The model under review builds one solid part; all positions refer to its coordinate system, in mm. A direction names the side the tool comes from. Round coordinates to 2 decimals unless told otherwise and drop trailing zeros. Order: outer loops, then holes, each group sorted by start corner. A loop starts at its lowest first (then second) coordinate and runs counter-clockwise, first axis right, second up. Notation, with made-up numbers: (26.5, 48) -> (42.5, 48) arc R22 cw to (42.5, 60) -> close; hole circle Ø11 at (32, -31). An arc over 180 degrees is marked (long way). Use a Markdown table: item, result. Add a question column.
```python
from build123d import *

# Parameters (mm, degrees)
CUT_EXTRUDE_1_DEPTH = 1.5
CHAMFER_1_SIZE      = 0.2


with BuildPart() as part:
    # 草图1 → 旋转1 (revolve)
    with BuildSketch(Plane(origin=(0, 0, 0), x_dir=(0, 0, -1), z_dir=(1, 0, 0)), mode=Mode.PRIVATE) as revolve_1_sk:
        Polygon((7, 0), (-7, 0), (-7, 1.9), (-6.7, 1.9), (-5.8, 1), (7, 1), align=None)
    revolve(revolve_1_sk.sketch.rotate(Axis((0, 0, -7), (0, 0, 1)), 90), axis=Axis((0, 0, -7), (0, 0, 1)))

    # 草图2 → 切除-拉伸1 (cut)
    with BuildSketch(Plane.XY.offset(7)):
        Polygon((0, 0.866025404), (-0.75, 0.433012702), (-0.75, -0.433012702), (0, -0.866025404), (0.75, -0.433012702), (0.75, 0.433012702), align=None)
    extrude(amount=-CUT_EXTRUDE_1_DEPTH, mode=Mode.SUBTRACT)

    # 倒角1
    chamfer_1_edges = [part.edges().sort_by_distance(p)[0] for p in [
        (1, 0, -7),
    ]]
    chamfer(chamfer_1_edges, length=CHAMFER_1_SIZE)


solid = part.part
```
Q1. For pin 1 (1.7 mm diameter, centred on x = 0, y = 0.5, fed in from +Z); pin 2 (2 mm diameter, centred on y = -1, z = -5, fed in from +X), all flat-tipped, find the tip position at first contact; note any pin that passes through.
Q2. Draft analysis for pull direction Y (two halves, no side actions). For faces 4 (the face through (1.9, -0.08, 6.85)), 5 (the face through (0, 0, -7)), 6 (the face through (-0.75, 0, 6)), state which applies: released by +Y, released by -Y, zero draft, split by the parting line, or undercut.
Q3. Add section B-B, the plane z = -1.75. Give the boundary of the cut face in (x, y), then the cut area to 3 significant figures.
Q4. Add section A-A, the plane y = 0. Give the boundary of the cut face in (x, z), then the cut area to 3 significant figures.
Q5. To check wall thickness, follow line 1 along Y through (x, z) = (-0.5, -0.5); line 2 along Y through (x, z) = (-0.6, -6.25); line 3 along X through (y, z) = (0.1, 6.25). State the ranges of each line that lie inside material, in increasing order.
Q6. For faces 1 (the face through (0, 0, 5.5)), 2 (the face through (1, 0, 7)), 3 (the face through (0, 1, -1)), list the 3-axis set-ups (+Z, -Z, +X, -X, +Y, -Y) from which the entire face can be reached by the end or side of a thin tool; tool diameter is ignored.
Return value:
| question | item | result |
|---|---|---|
| 1 | pin 1 | z = 7 |
| 1 | pin 2 | x = 1 |
| 2 | face 4 | split by the parting line |
| 2 | face 5 | zero draft |
| 2 | face 6 | undercut |
| 3 | outline | circle Ø2 at (0, 0) |
| 3 | area | 3.14 mm² |
| 4 | outline | (-1.9, 6.7) -> (-1, 5.8) -> (-1, -6.8) -> (-0.8, -7) -> (0.8, -7) -> (1, -6.8) -> (1, 5.8) -> (1.9, 6.7) -> (1.9, 7) -> (0.75, 7) -> (0.75, 5.5) -> (-0.75, 5.5) -> (-0.75, 7) -> (-1.9, 7) -> close |
| 4 | area | 27.1 mm² |
| 5 | line 1 | -0.87 to 0.87 |
| 5 | line 2 | -0.8 to 0.8 |
| 5 | line 3 | -1.45 to -0.75, 0.75 to 1.45 |
| 6 | face 1 | +Z |
| 6 | face 2 | +Z, +X, -X, +Y, -Y |
| 6 | face 3 | -Z |
